For this review, use the dimensioned drawing (mm, ordinates from the lowest corner) and the shaded views. A direction names the side the tool comes from. Give positions to 0.01 mm unless a question says otherwise; leave off trailing zeros. Loops run counter-clockwise (first coordinate to the right, second up) from the corner with the lowest first, then second, coordinate; pieces in that order, holes last. Notation, with made-up numbers: M -27,49.5 L -7,49.5 A14 ccw -7,58.5 Z; hole C 8.25,35 d9. An arc over 180 degrees is marked long. Use one line per item in the form item = value. Start each with the question number.
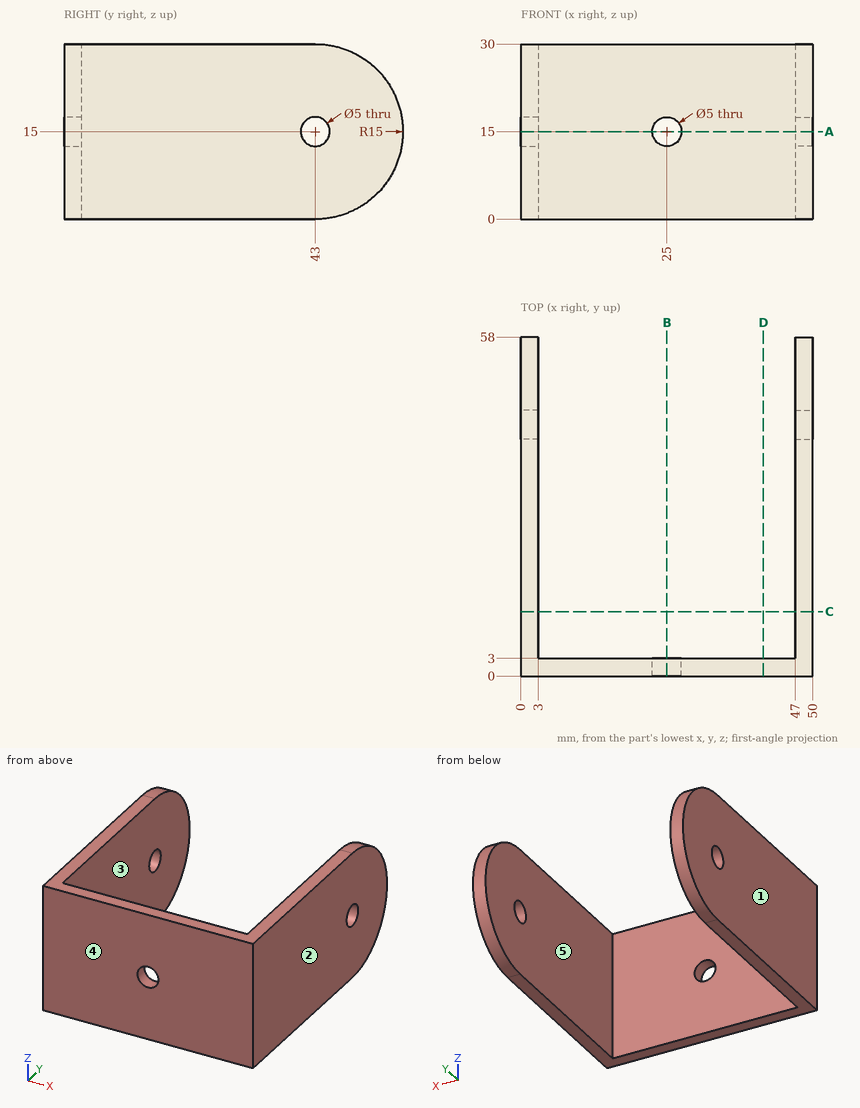
Q1. For the marked faces 4 and 5, list the 3-axis set-ups (+Z, -Z, +X, -X, +Y, -Y) from which the entire face can be reached by the end or side of a thin tool; tool diameter is ignored.
Q2. Take a section at D-D on x = 41.5. Give the boundary of the cut face in (y, z), plus the area to 3 significant figures.
Q3. Take a section at C-C on y = 11. Give the boundary of the cut face in (x, z), plus the area to 3 significant figures.
Q4. The part is to be moulded in two halves that separate along X. For the marked faces 1, 2 and 3, say which applies: pulls with the +X half, pulls with the -X half, needs draft (parallel to the pull), parting line crosses it, or undercut.
Q5. Take a section at B-B on x = 25. Give the boundary of the cut face in (y, z), plus the area to 3 significant figures.
Q6. Wall thickness on probe 1 along X at (y, z) = (34, 8); probe 2 along Y at (x, z) = (1.75, 15); probe 3 along Y at (x, z) = (31.5, 3): over which ranges is each line inside the solid? List them lowest first.
Q7. Clearance check with a flat-ended pin moving along its axis: pin 1 Ø5 at (x, z) = (44, 20.5) entering from +Y. State where the tip first meets the part, or that it passes through.
Q8. Take a section at A-A on z = 15. Give the boundary of the cut face in (x, y), plus the area to 3 significant figures.
Response values:
q1.face_4 = +Z, -Z, +X, -X, -Y
q1.face_5 = +Z, -Z, +Y
q2.outline = M 0,0 L 3,0 L 3,30 L 0,30 Z
q2.area = 90.0 mm^2
q3.outline = M 0,0 L 3,0 L 3,30 L 0,30 Z; M 47,0 L 50,0 L 50,30 L 47,30 Z
q3.area = 180 mm^2
q4.face_1 = pulls with the -X half
q4.face_2 = pulls with the +X half
q4.face_3 = undercut
q5.outline = M 0,0 L 3,0 L 3,12.5 L 0,12.5 Z; M 0,17.5 L 3,17.5 L 3,30 L 0,30 Z
q5.area = 75.0 mm^2
q6.probe_1 = 0 to 3, 47 to 50
q6.probe_2 = 0 to 40.5, 45.5 to 58
q6.probe_3 = 0 to 3
q7.pin_1 = 3
q8.outline = M 0,0 L 22.5,0 L 22.5,3 L 3,3 L 3,40.5 L 0,40.5 Z; M 0,45.5 L 3,45.5 L 3,58 L 0,58 Z; M 27.5,0 L 50,0 L 50,40.5 L 47,40.5 L 47,3 L 27.5,3 Z; M 47,45.5 L 50,45.5 L 50,58 L 47,58 Z
q8.area = 435 mm^2
